```python
from build123d import *

# Parameters (mm, degrees)
ESQUISSE1_R             = 15
BOSS_EXTRU_1_DEPTH      = 100
ESQUISSE2_R             = 15
ENL_V_MAT_EXTRU_1_DEPTH = 590.067059001
CONG_1_R                = 10


with BuildPart() as part:
    # Esquisse1 → Boss.-Extru.1 (new body)
    with BuildSketch(Plane.XY):
        with BuildLine():
            Line((10, 0), (190.505102572, 0))
            ThreePointArc((190.505102572, 0), (215, -20), (239.494897428, 0))
            Line((239.494897428, 0), (420, 0))
            Line((420, 0), (430, 0))
            Line((430, 0), (430, 390))
            Line((430, 390), (420, 390))
            Line((420, 390), (420, 10))
            Line((420, 10), (239.494897428, 10))
            ThreePointArc((239.494897428, 10), (215, 30), (190.505102572, 10))
            Line((190.505102572, 10), (10, 10))
            Line((10, 10), (10, 390))
            Line((10, 390), (0, 390))
            Line((0, 390), (0, 0))
            Line((0, 0), (10, 0))
        make_face()
        with Locations((215, 5)):
            Circle(ESQUISSE1_R, mode=Mode.SUBTRACT)
    extrude(amount=BOSS_EXTRU_1_DEPTH)

    # Esquisse2 → Enlèv. mat.-Extru.1 (cut, through all)
    with BuildSketch(Plane(origin=(430, 0, 0), x_dir=(0, 0, -1), z_dir=(1, 0, 0))):
        with BuildLine():
            Line((-100, 305), (-78.45468447, 369.504258609))
            ThreePointArc((-78.45468447, 369.504258609), (-67.533856417, 384.342635008), (-50, 390))
            Line((-50, 390), (-100, 390))
            Line((-100, 390), (-100, 305))
        make_face()
        Polygon((-120.94696684, 305), (-100, 305), (-100, 390), (-50, 390), (0, 390), (0, 305), (20.94696684, 305), (20.94696684, 555.583179512), (-120.94696684, 555.583179512), align=None)
        with BuildLine():
            Line((0, 390), (-50, 390))
            ThreePointArc((-50, 390), (-32.466143583, 384.342635008), (-21.54531553, 369.504258609))
            Line((-21.54531553, 369.504258609), (0, 305))
            Line((0, 305), (0, 390))
        make_face()
        with Locations(Location((-50, 360, 0), (0, 0, 90))):
            Circle(ESQUISSE2_R)
    extrude(amount=-ENL_V_MAT_EXTRU_1_DEPTH, mode=Mode.SUBTRACT)

    # Congé1
    cong_1_edges = [part.edges().sort_by_distance(p)[0] for p in [
        (0, 0, 50),
        (10, 10, 50),
        (190.505102572, 10, 50),
        (239.494897428, 10, 50),
        (420, 10, 50),
        (430, 0, 50),
        (239.494897428, 0, 50),
        (190.505102572, 0, 50),
        (425, 305, 0),
        (425, 305, 100),
        (5, 305, 100),
        (5, 305, 0),
    ]]
    fillet(cong_1_edges, radius=CONG_1_R)


solid = part.part
```
Geometry check sheet. Reference: the model listing, model coordinates, mm. A direction names the side the tool comes from. Give positions to 0.01 mm unless a question says otherwise; leave off trailing zeros. Order: outer loops, then holes, each group sorted by start corner. A loop starts at its lowest first (then second) coordinate and runs counter-clockwise, first axis right, second up.
1. Section check D-D, the plane y = 360. Enter the section's corners in (x, z).
2. Access from +Z, -Z, +X, -X, +Y, -Y to the whole of each face (thin tool, end or side, straight path). Record for faces 1 (the face through (332, 0, 49)), 2 (the face through (214, 23, 0)), 3 (the face through (329, 10, 49)).
3. Section check B-B, the plane y = 100. Enter the section's corners in (x, z), and give its area (3 significant figures).
4. Thickness scan on L1, parallel to X at y = 96, z = 50; L2, parallel to Y at x = 23, z = 95.5; L3, parallel to Z at x = 424.75, y = 360. Record the ranges inside material, lowest first.
5. Section check A-A, the plane x = 215. Enter the section's corners in (y, z).
6. Release check for a two-part mould opening along X. For faces 4 (the face through (12.85, 13.01, 50.7)), 5 (the face through (215, -20, 49)), 6 (the face through (425.07, 374.307, 54.506)) record: pulls with the +X half, pulls with the -X half, needs draft (parallel to the pull), parting line crosses it, or undercut.
7. Gauge pin test, flat ends, axial feed: pin 1 Ø10 at (x, z) = (94.5, 26) entering from -Y; pin 2 Ø3 at (x, z) = (137.5, 23) entering from +Y; pin 3 Ø3 at (x, z) = (193, 31.5) entering from -Y; pin 4 Ø24 at (y, z) = (360, 50) entering from +X. Record the tip position at first contact, or that the pin passes through.
8. Section check C-C, the plane z = 55. Give the number of separate pieces and of enclosed holes in the cut face, and give its area (3 significant figures).
Values follow:
1. outline: (0, 18.37) - (10, 18.37) - (10, 35) - (0, 35) - close; (0, 65) - (10, 65) - (10, 81.63) - (0, 81.63) - close; (420, 18.37) - (430, 18.37) - (430, 35) - (420, 35) - close; (420, 65) - (430, 65) - (430, 81.63) - (420, 81.63) - close
2. face 1: +Z, -Z, +X, -Y
2. face 2: -Z, +X, -X, +Y, -Y
2. face 3: +Z, -Z, +Y
3. outline: (0, 0) - (10, 0) - (10, 100) - (0, 100) - close; (420, 0) - (430, 0) - (430, 100) - (420, 100) - close
3. area: 2,000 mm2
4. L1: x = 0 to 10, 420 to 430
4. L2: y = 0 to 10
4. L3: z = 18.37 to 35, 65 to 81.63
5. outline: (-20, 0) - (-10, 0) - (-10, 100) - (-20, 100) - close; (20, 0) - (30, 0) - (30, 100) - (20, 100) - close
6. face 4: undercut
6. face 5: parting line crosses it
6. face 6: needs draft
7. pin 1: stops at y = 0
7. pin 2: stops at y = 10
7. pin 3: stops at y = -9.31
7. pin 4: passes through
8. separate pieces: 3
8. enclosed holes: 1
8. area: 12,100 mm2
